from build123d import *

# Parameters (mm, degrees)
F0_W     = 55
F0_H     = 40
F1_DEPTH = 50.1
F2_SIZE  = 20
F4_D     = 4.2
F5_SIZE  = 1


with BuildPart() as f1:
    # F0 (on Top) → F1 (new body)
    with BuildSketch(Plane.XY):
        with Locations((27.5, 20)):
            Rectangle(F0_W, F0_H)
    extrude(amount=F1_DEPTH)

    # F2
    f2_edges = [f1.edges().sort_by_distance(p)[0] for p in [
        (27.5, 0, 50.1),
    ]]
    chamfer(f2_edges, length=F2_SIZE)

    # F4 (through all)
    with Locations(Plane(origin=(0, -15.05, 15.05), x_dir=(1, 0, 0), z_dir=(0, -0.7071067812, 0.7071067812))):
        with Locations((40, 38.7047119439), (15, 38.7047119439)):
            Hole(F4_D / 2)

    # F5
    f5_edges = [f1.edges().sort_by_distance(p)[0] for p in [
        (27.5, 40, 50.1),
    ]]
    chamfer(f5_edges, length=F5_SIZE)


solid = f1.part
CAD build for the part. Positions are in the model's coordinates, mm. Coordinates: 2 decimals unless noted, no trailing zeros. Loops run counter-clockwise (first coordinate to the right, second up) from the corner with the lowest first, then second, coordinate; pieces in that order, holes last. Notation, with made-up numbers: (11.5, 27) -> (50.5, 27) arc R18 cw to (50.5, 62) -> close; hole circle Ø3 at (-1, 77.5). An arc over 180 degrees is marked (long way). One line per item, written item: value.
1. Slice it at D-D on z = 34. Give the number of separate pieces and of enclosed holes in the cut face, and give its area (3 significant figures).
Answers:
separate pieces: 1
enclosed holes: 2
area: 1,950 mm^2
2. Slice it at B-B on z = 46.5. Write the cut outline in (x, y), and give its area (3 significant figures).
Answers:
outline: (0, 16.4) -> (55, 16.4) -> (55, 40) -> (0, 40) -> close
area: 1,300 mm^2
3. Flat gauge pins, fed straight in: P1, Ø12, axis at x = 34, z = 35, coming from the -Y side; P2, Ø6, axis at x = 44.5, z = 37, coming from the -Y side. Where does each tip first touch, or does it go through?
Answers:
P1: stops at y = 0
P2: stops at y = 3.9
4. Slice it at A-A on x = 4. Write the cut outline in (y, z).
Answers:
outline: (0, 0) -> (40, 0) -> (40, 49.1) -> (39, 50.1) -> (20, 50.1) -> (0, 30.1) -> close
5. Pull direction X, two halves, no side cores. Call faces 1 (the face through (40.455, 25.674, 26.163)), 2 (the face through (27, 30, 50.1)), 3 (the face through (0, 20, 25)), 4 (the face through (15.455, 25.674, 26.163)): pulls with the +X half, pulls with the -X half, needs draft (parallel to the pull), parting line crosses it, or undercut.
Answers:
face 1: undercut
face 2: needs draft
face 3: pulls with the -X half
face 4: undercut
6. Drill centre lines: line 1 (X direction, y = 26, z = 26); line 2 (Y direction, x = 13, z = 43); line 3 (Z direction, x = 14.5, y = 26). Where is each one in solid material? Low to high. Write a range as [from, to].
Answers:
line 1: x = [0, 14.18], [15.82, 39.18], [40.82, 55]
line 2: y = [12.9, 40]
line 3: z = [0, 25.85], [31.62, 50.1]
7. Slice it at C-C on y = 4. Write the cut outline in (x, z), and give its area (3 significant figures).
Answers:
outline: (0, 0) -> (55, 0) -> (55, 34.1) -> (0, 34.1) -> close
area: 1,880 mm^2
